Here's how the part is built. I have some questions about the finished solid (model axes, mm). A direction names the side the tool comes from. Coordinates: 2 decimals unless noted, no trailing zeros. Write each loop counter-clockwise with the first axis right and the second up, starting at its lowest first coordinate (ties: lowest second). Pieces come first, ordered by that corner, then holes. Notation, with made-up numbers: (-27, 66.5) -> (6, 66.5) arc R27 cw to (6, 105.5) -> close; hole circle Ø11 at (34.5, -1). An arc over 180 degrees is marked (long way). Put each result on its own line as item: value. Start each with the question number.
Item 1: I want a section at B-B, the plane x = 0. List the corners of the cut face in (y, z) for me.
Item 2: On a 3-axis mill with a long thin cutter (end or side, diameter ignored), from which of +Z, -Z, +X, -X, +Y, -Y can I reach the whole of each face in a straight line? I mean faces 1 (the face through (0, -10, -41)), 2 (the face through (6, -12, 48)). Say none if no direction works.
Item 3: I want a section at C-C, the plane z = -3.5. List the corners of the cut face in (x, y) for me.
Item 4: I need wall thicknesses on line 1 (Z direction, x = 0, y = -1.75); line 2 (Z direction, x = 1.5, y = -2.25); line 3 (Y direction, x = -4.5, z = 12). Which ranges of each line are inside material? Lowest first, please. Write a range as [from, to].
Item 5: I want a section at A-A, the plane y = -6.25. List the corners of the cut face in (x, z) for me.
Item 6: If we mould it in two halves opening along Z, with no side actions, what happens to faces 3 (the face through (0, -10, 41)), 4 (the face through (0, -13, 50)), 5 (the face through (0, -12, -50))? For each: released by +Z, released by -Z, zero draft, split by the parting line, or undercut.
from build123d import *

# Parameters (mm, degrees)
F3_DEPTH = 3
F4_DEPTH = 3


with BuildPart() as f2:
    # F2: sweep along a path in F0
    with BuildLine(Plane.YZ) as f2_path:
        Line((0, 47), (-25, 47))
        Line((-25, 47), (-25, -47))
        Line((-25, -47), (0, -47))
    # F1 (on Front) → F2 (sweep)
    with BuildSketch(Plane.XZ):
        with BuildLine():
            Line((6, 47), (-6, 47))
            ThreePointArc((-6, 47), (0, 41), (6, 47))
        make_face()
    sweep(path=f2_path.line, transition=Transition.RIGHT)

    # F3 (add): a face of the model
    f3_faces = [f2.faces().sort_by_distance(p)[0] for p in [
        (0, -12.5, 47),
    ]]
    extrude(f3_faces, amount=F3_DEPTH)

    # F4 (add): a face of the model
    f4_faces = [f2.faces().sort_by_distance(p)[0] for p in [
        (0, -12.5, -47),
    ]]
    extrude(f4_faces, amount=F4_DEPTH)


solid = f2.part
Calculated:
1. outline: (-25, -50) -> (0, -50) -> (0, -41) -> (-19, -41) -> (-19, 41) -> (0, 41) -> (0, 50) -> (-25, 50) -> close
2. face 1: +Y
2. face 2: +Z, -Z, +X, +Y, -Y
3. outline: (-6, -25) -> (6, -25) arc R6 ccw to start
4. line 1: z = [-50, -41], [41, 50]
4. line 2: z = [-50, -41.19], [41.19, 50]
4. line 3: y = [-25, -21.03]
5. outline: (-6, -50) -> (6, -50) -> (6, -47) arc R6 ccw to (-6, -47) -> close; (-6, 47) arc R6 ccw to (6, 47) -> (6, 50) -> (-6, 50) -> close
6. face 3: undercut
6. face 4: released by +Z
6. face 5: released by -Z
